Check sheet for the modelled part. Datum: model origin and axes. Units: mm. Face numbers are marked on the shaded views. Coordinates: 2 decimals unless noted, no trailing zeros. Write each loop counter-clockwise with the first axis right and the second up, starting at its lowest first coordinate (ties: lowest second). Pieces come first, ordered by that corner, then holes. Notation, with made-up numbers: M 27,-38 L 50,-38 A15 cw 50,-20 Z; hole C -12.75,78 d4. An arc over 180 degrees is marked long. Answer as CSV lines item,"result". Start each with the question number.
Q1. Thickness scan on line 1 along X through (y, z) = (0, 8); line 2 along Y through (x, z) = (-11.5, 3.25); line 3 along Y through (x, z) = (12, 3.75). Record the ranges inside material, lowest first. Write a range as from..to.
Q2. Mould release check, pull along X, two halves, no side actions. Record for the marked faces 1, 2, 3 and 4: pulls with the +X half, pulls with the -X half, needs draft (parallel to the pull), parting line crosses it, or undercut.
Q3. Sectioned sample at D-D, the plane x = -1.5. Record the cut outline in (y, z).
Q4. Sectioned sample at A-A, the plane y = -4.5. Record the cut outline in (x, z).
Q5. Sectioned sample at B-B, the plane x = -6.25. Record the cut outline in (y, z).
Q6. Sectioned sample at C-C, the plane z = 4. Record the cut outline in (x, y), then the cut area to 3 significant figures.
Q7. Depth check by flat-ended pin: pin 1 Ø1.5 at (x, y) = (-7.5, -10) entering from -Z; pin 2 Ø0.5 at (x, z) = (-12.5, 0.5) entering from +Y; pin 3 Ø8.5 at (x, y) = (-1, -4) entering from +Z. Enter the tip coordinate at first touch or a pass-through.
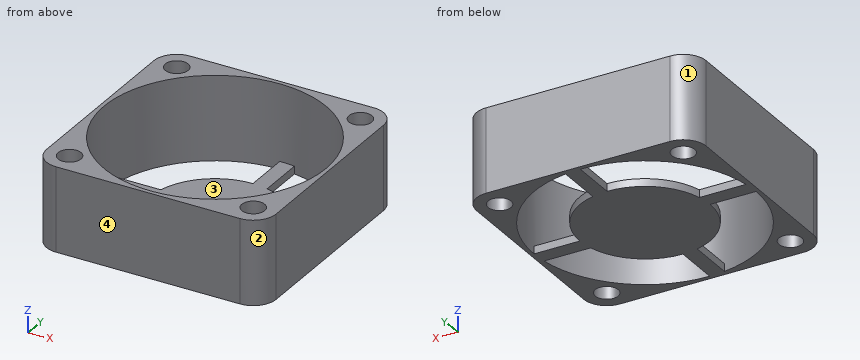
from build123d import *

# Parameters (mm, degrees)
F0_R     = 1.5
F0_R_2   = 14.5
F1_DEPTH = 11
F3_DEPTH = 1


with BuildPart() as f1:
    # F0 (on Top) → F1 (new body)
    with BuildSketch(Plane.XY):
        with BuildLine():
            Line((-12, -15), (12, -15))
            ThreePointArc((12, -15), (14.12132, -14.12132), (15, -12))
            Line((15, -12), (15, 12))
            ThreePointArc((15, 12), (14.12132, 14.12132), (12, 15))
            Line((12, 15), (-12, 15))
            ThreePointArc((-12, 15), (-14.12132, 14.12132), (-15, 12))
            Line((-15, 12), (-15, -12))
            ThreePointArc((-15, -12), (-14.12132, -14.12132), (-12, -15))
        make_face()
        with Locations((-12, -12)):
            Circle(F0_R, mode=Mode.SUBTRACT)
        with Locations((12, -12)):
            Circle(F0_R, mode=Mode.SUBTRACT)
        Circle(F0_R_2, mode=Mode.SUBTRACT)
        with Locations((-12, 12)):
            Circle(F0_R, mode=Mode.SUBTRACT)
        with Locations((12, 12)):
            Circle(F0_R, mode=Mode.SUBTRACT)
    extrude(amount=F1_DEPTH)

    # F2 (on face) → F3 (join)
    with BuildSketch(Plane(origin=(0, 0, 0), x_dir=(1, 0, 0), z_dir=(0, 0, -1))):
        with BuildLine():
            Line((2, -15), (2, -8.261356))
            ThreePointArc((2, -8.261356), (6.680195, -5.255949), (8.5, 0))
            Line((8.5, 0), (15, 0))
            Line((15, 0), (15, 2))
            Line((15, 2), (8.261356, 2))
            ThreePointArc((8.261356, 2), (5.255949, 6.680195), (0, 8.5))
            Line((0, 8.5), (0, 15))
            Line((0, 15), (-2, 15))
            Line((-2, 15), (-2, 8.261356))
            ThreePointArc((-2, 8.261356), (-6.680195, 5.255949), (-8.5, 0))
            Line((-8.5, 0), (-15, 0))
            Line((-15, 0), (-15, -2))
            Line((-15, -2), (-8.261356, -2))
            ThreePointArc((-8.261356, -2), (-5.255949, -6.680195), (0, -8.5))
            Line((0, -8.5), (0, -15))
            Line((0, -15), (2, -15))
        make_face()
    extrude(amount=-F3_DEPTH)


solid = f1.part
Output:
1,line 1,"x = -15..-14.5, 14.5..15"
1,line 2,"y = -15..-13.41, -10.59..-8.83, 8.83..10.59, 13.41..15"
1,line 3,"y = -15..-13.5, -10.5..-8.14, 8.14..10.5, 13.5..15"
2,face 1,"pulls with the -X half"
2,face 2,"pulls with the +X half"
2,face 3,"undercut"
2,face 4,"needs draft"
3,outline,"M -15,0 L 8.37,0 L 8.37,1 L -14.42,1 L -14.42,11 L -15,11 Z; M 14.42,0 L 15,0 L 15,11 L 14.42,11 Z"
4,outline,"M -15,0 L -13.78,0 L -13.78,11 L -15,11 Z; M -7.21,0 L 7.21,0 L 7.21,1 L -7.21,1 Z; M 13.78,0 L 15,0 L 15,11 L 13.78,11 Z"
5,outline,"M -15,0 L -13.08,0 L -13.08,11 L -15,11 Z; M -5.76,0 L 5.76,0 L 5.76,1 L -5.76,1 Z; M 13.08,0 L 15,0 L 15,11 L 13.08,11 Z"
6,outline,"M -15,-12 A3 ccw -12,-15 L 12,-15 A3 ccw 15,-12 L 15,12 A3 ccw 12,15 L -12,15 A3 ccw -15,12 Z; hole C 0,0 d29; hole C -12,-12 d3; hole C -12,12 d3; hole C 12,-12 d3; hole C 12,12 d3"
6,area,"203 mm^2"
7,pin 1,"passes through"
7,pin 2,"stops at y = 14.99"
7,pin 3,"stops at z = 1"
